Could you check a few things on this model? Use its own coordinates, in mm. A direction names the side the tool comes from. Give positions to 0.01 mm unless a question says otherwise; leave off trailing zeros. Loops run counter-clockwise (first coordinate to the right, second up) from the corner with the lowest first, then second, coordinate; pieces in that order, holes last. Notation, with made-up numbers: (-23.5, 71) -> (8.5, 71) arc R17 ccw to (8.5, 103) -> close; hole circle Ø7 at (77, 20). An arc over 180 degrees is marked (long way). Write each question's results on one line, items separated by ' | '. Start each with the question number.
Q1. Will these pins go through, and if not, where does the flat tip stop? P1, Ø4, axis at x = -31, y = -34.5, coming from the -Z side (3 decimals); P2, Ø6, axis at x = -31.75, z = -66.675, coming from the -Y side; P3, Ø8.5, axis at x = 34.75, z = 39.195, coming from the -Y side; P4, Ø20.5, axis at x = 0, z = 4.445, coming from the +Y side.
Q2. If we section it at C-C, the plane z = 11: List the corners of the cut face in (x, y) for me (3 decimals).
Q3. If we section it at A-A, the plane x = 0: List the corners of the cut face in (y, z) for me (3 decimals), plus the area to 3 significant figures.
Q4. If I drill on line 1 along X through (y, z) = (-38.5, 11) (3 decimals); line 2 along Y through (x, z) = (-9.5, 18.5); line 3 along Z through (x, y) = (-5.5, -17) (3 decimals), over which ranges is the centre line in solid material (lowest first)?
Q5. If we section it at B-B, the plane y = -6.5: List the corners of the cut face in (x, z) for me (3 decimals), plus the area to 3 significant figures.
Q6. If we section it at D-D, the plane y = -35: List the corners of the cut face in (x, z) for me (3 decimals), plus the area to 3 significant figures.
Q7. We'd pull the mould along X, two halves only. Please class faces 1 (the face through (-45.371, -51.333, 3.84)), 2 (the face through (3.81, 3.52, 16.56)), 3 (the face through (47.625, -31, -51)): released by +X, released by -X, zero draft, split by the parting line, or undercut.
Q8. Which directions (+Z, -Z, +X, -X, +Y, -Y) give clear straight access to the entire face, cutting with the end or side of a thin tool? Please do faces 4 (the face through (-37.28, 2.46, -31.85)), 5 (the face through (1, 2, -12)), 6 (the face through (-43.18, -41, 1)), 7 (the face through (-1, -30, -82)), 8 (the face through (45.43, -55.17, -35.09)).
from build123d import *

# Parameters (mm, degrees)
SKETCH1_W                      = 95.25
SKETCH1_H                      = 63.5
SKETCH1_H_2                    = 95.25
BOSS_EXTRUDE1_DEPTH            = 5
BOSS_EXTRUDE2_DEPTH            = 88.9
CUT_EXTRUDE1_REACH             = 170.812
CUT_EXTRUDE1_DIRECTION_2_REACH = 170.812
SKETCH4_R                      = 37.5
CUT_EXTRUDE2_DEPTH             = 2
CUT_EXTRUDE3_REACH             = 170.812
CUT_EXTRUDE3_DIRECTION_2_REACH = 170.812
FILLET1_R                      = 6.35
SKETCH6_W                      = 95.25
SKETCH6_H                      = 57.15
BOSS_EXTRUDE3_DEPTH            = 30
CUT_EXTRUDE4_REACH             = 136.485
SKETCH7_R                      = 2.665000004
CUT_EXTRUDE5_REACH             = 155.082
SKETCH8_R                      = 12.7
CUT_EXTRUDE6_REACH             = 152.067
SKETCH9_R                      = 3.25


with BuildPart() as part:
    # Sketch1 → Boss-Extrude1 (new body)
    with BuildSketch(Plane(origin=(0, 0, 0), x_dir=(1, 0, 0), z_dir=(0, 1, 0))):
        with Locations((0, 79.375)):
            Rectangle(SKETCH1_W, SKETCH1_H)
        Rectangle(SKETCH1_W, SKETCH1_H_2)
    extrude(amount=BOSS_EXTRUDE1_DEPTH)

    # Sketch2 → Boss-Extrude2 (add)
    with BuildSketch(Plane(origin=(0, 0, 0), x_dir=(-1, 0, 0), z_dir=(0, -1, 0))):
        Polygon((43.18, 38.735), (43.18, -47.625), (47.625, -47.625), (47.625, 53.975), (-47.625, 53.975), (-47.625, -47.625), (-43.18, -47.625), (-43.18, 38.735), align=None)
    extrude(amount=BOSS_EXTRUDE2_DEPTH)

    # Sketch3 → Cut-Extrude1 (cut, up to next)
    with BuildSketch(Plane.ZY.offset(-43.18), mode=Mode.PRIVATE) as cut_extrude1_sk1:
        Polygon((-38.735, -88.9), (47.625, -12.7), (47.625, -88.9), align=None)
    cut_extrude1_tool1 = extrude(cut_extrude1_sk1.sketch, amount=-CUT_EXTRUDE1_REACH, mode=Mode.PRIVATE) & part.part
    add(cut_extrude1_tool1.solids().sort_by_distance((43.18, -63.5, 18.838333))[0], mode=Mode.SUBTRACT)

    # Sketch3 → Cut-Extrude1 direction 2 (cut, up to next)
    with BuildSketch(Plane.ZY.offset(-43.18), mode=Mode.PRIVATE) as cut_extrude1_direction_2_sk1:
        Polygon((-38.735, -88.9), (47.625, -12.7), (47.625, -88.9), align=None)
    cut_extrude1_direction_2_tool1 = extrude(cut_extrude1_direction_2_sk1.sketch, amount=CUT_EXTRUDE1_DIRECTION_2_REACH, mode=Mode.PRIVATE) & part.part
    add(cut_extrude1_direction_2_tool1.solids().sort_by_distance((43.18, -63.5, 18.838333))[0], mode=Mode.SUBTRACT)

    # Sketch4 → Cut-Extrude2 (cut)
    with BuildSketch(Plane(origin=(0, 0, 0), x_dir=(-1, 0, 0), z_dir=(0, -1, 0))):
        with Locations(Location((0, -4.445, 0), (0, 0, 90))):
            Circle(SKETCH4_R)
    extrude(amount=-CUT_EXTRUDE2_DEPTH, mode=Mode.SUBTRACT)

    # Sketch5 → Cut-Extrude3 (cut, up to next)
    with BuildSketch(Plane(origin=(-43.18, 0, 0), x_dir=(0, 0, -1), z_dir=(1, 0, 0)), mode=Mode.PRIVATE) as cut_extrude3_sk1:
        Polygon((38.735, 0), (-33.225441849, 0), (38.735, -63.494507514), align=None)
    cut_extrude3_tool1 = extrude(cut_extrude3_sk1.sketch, amount=-CUT_EXTRUDE3_REACH, mode=Mode.PRIVATE) & part.part
    add(cut_extrude3_tool1.solids().sort_by_distance((-43.18, -21.164836, -14.748186))[0], mode=Mode.SUBTRACT)

    # Sketch5 → Cut-Extrude3 direction 2 (cut, up to next)
    with BuildSketch(Plane(origin=(-43.18, 0, 0), x_dir=(0, 0, -1), z_dir=(1, 0, 0)), mode=Mode.PRIVATE) as cut_extrude3_direction_2_sk1:
        Polygon((38.735, 0), (-33.225441849, 0), (38.735, -63.494507514), align=None)
    cut_extrude3_direction_2_tool1 = extrude(cut_extrude3_direction_2_sk1.sketch, amount=CUT_EXTRUDE3_DIRECTION_2_REACH, mode=Mode.PRIVATE) & part.part
    add(cut_extrude3_direction_2_tool1.solids().sort_by_distance((-43.18, -21.164836, -14.748186))[0], mode=Mode.SUBTRACT)

    # Fillet1
    fillet1_edges = [part.edges().sort_by_distance(p)[0] for p in [
        (45.4025, -63.494507514, -38.735),
        (45.4025, 0, 33.225441849),
        (-45.4025, 0, 33.225441849),
        (-45.4025, -63.494507514, -38.735),
    ]]
    fillet(fillet1_edges, radius=FILLET1_R)

    # Sketch6 → Boss-Extrude3 (add)
    with BuildSketch(Plane.XZ):
        with Locations((0, -82.55)):
            Rectangle(SKETCH6_W, SKETCH6_H)
    extrude(amount=BOSS_EXTRUDE3_DEPTH)

    # Sketch7 → Cut-Extrude4 (cut, up to next)
    with BuildSketch(Plane(origin=(0, -30, 0), x_dir=(-1, 0, 0), z_dir=(0, -1, 0)), mode=Mode.PRIVATE) as cut_extrude4_sk1:
        with Locations(Location((0, 97.872945695, 0), (0, 0, 90))):
            Circle(SKETCH7_R)
    cut_extrude4_tool1 = extrude(cut_extrude4_sk1.sketch, amount=-CUT_EXTRUDE4_REACH, mode=Mode.PRIVATE) & part.part
    # Sketch7 → Cut-Extrude4 (cut, up to next)
    with BuildSketch(Plane(origin=(0, -30, 0), x_dir=(-1, 0, 0), z_dir=(0, -1, 0)), mode=Mode.PRIVATE) as cut_extrude4_sk2:
        with Locations(Location((31.75, 66.675, 0), (0, 0, 90))):
            Circle(SKETCH7_R)
    cut_extrude4_tool2 = extrude(cut_extrude4_sk2.sketch, amount=-CUT_EXTRUDE4_REACH, mode=Mode.PRIVATE) & part.part
    # Sketch7 → Cut-Extrude4 (cut, up to next)
    with BuildSketch(Plane(origin=(0, -30, 0), x_dir=(-1, 0, 0), z_dir=(0, -1, 0)), mode=Mode.PRIVATE) as cut_extrude4_sk3:
        with Locations(Location((-31.75, 66.675, 0), (0, 0, 90))):
            Circle(SKETCH7_R)
    cut_extrude4_tool3 = extrude(cut_extrude4_sk3.sketch, amount=-CUT_EXTRUDE4_REACH, mode=Mode.PRIVATE) & part.part
    add(cut_extrude4_tool1.solids().sort_by_distance((0, -30, -97.872946))[0], mode=Mode.SUBTRACT)
    add(cut_extrude4_tool2.solids().sort_by_distance((-31.75, -30, -66.675))[0], mode=Mode.SUBTRACT)
    add(cut_extrude4_tool3.solids().sort_by_distance((31.75, -30, -66.675))[0], mode=Mode.SUBTRACT)

    # Sketch8 → Cut-Extrude5 (cut, up to next)
    with BuildSketch(Plane(origin=(0, 5, 0), x_dir=(1, 0, 0), z_dir=(0, 1, 0)), mode=Mode.PRIVATE) as cut_extrude5_sk1:
        with Locations(Location((0, -4.445, 0), (0, 0, 270))):
            Circle(SKETCH8_R)
    cut_extrude5_tool1 = extrude(cut_extrude5_sk1.sketch, amount=-CUT_EXTRUDE5_REACH, mode=Mode.PRIVATE) & part.part
    add(cut_extrude5_tool1.solids().sort_by_distance((0, 5, 4.445))[0], mode=Mode.SUBTRACT)

    # Sketch9 → Cut-Extrude6 (cut, up to next)
    with BuildSketch(Plane(origin=(0, 0, 0), x_dir=(-1, 0, 0), z_dir=(0, -1, 0)), mode=Mode.PRIVATE) as cut_extrude6_sk1:
        with Locations(Location((34.75, -39.195, 0), (0, 0, 90))):
            Circle(SKETCH9_R)
    cut_extrude6_tool1 = extrude(cut_extrude6_sk1.sketch, amount=-CUT_EXTRUDE6_REACH, mode=Mode.PRIVATE) & part.part
    # Sketch9 → Cut-Extrude6 (cut, up to next)
    with BuildSketch(Plane(origin=(0, 0, 0), x_dir=(-1, 0, 0), z_dir=(0, -1, 0)), mode=Mode.PRIVATE) as cut_extrude6_sk2:
        with Locations(Location((-34.75, -39.195, 0), (0, 0, 90))):
            Circle(SKETCH9_R)
    cut_extrude6_tool2 = extrude(cut_extrude6_sk2.sketch, amount=-CUT_EXTRUDE6_REACH, mode=Mode.PRIVATE) & part.part
    # Sketch9 → Cut-Extrude6 (cut, up to next)
    with BuildSketch(Plane(origin=(0, 0, 0), x_dir=(-1, 0, 0), z_dir=(0, -1, 0)), mode=Mode.PRIVATE) as cut_extrude6_sk3:
        with Locations(Location((34.396603139, 30.34702737, 0), (0, 0, 90))):
            Circle(SKETCH9_R)
    cut_extrude6_tool3 = extrude(cut_extrude6_sk3.sketch, amount=-CUT_EXTRUDE6_REACH, mode=Mode.PRIVATE) & part.part
    # Sketch9 → Cut-Extrude6 (cut, up to next)
    with BuildSketch(Plane(origin=(0, 0, 0), x_dir=(-1, 0, 0), z_dir=(0, -1, 0)), mode=Mode.PRIVATE) as cut_extrude6_sk4:
        with Locations(Location((-34.75, 30.305, 0), (0, 0, 90))):
            Circle(SKETCH9_R)
    cut_extrude6_tool4 = extrude(cut_extrude6_sk4.sketch, amount=-CUT_EXTRUDE6_REACH, mode=Mode.PRIVATE) & part.part
    add(cut_extrude6_tool1.solids().sort_by_distance((-34.75, 0, 39.195))[0], mode=Mode.SUBTRACT)
    add(cut_extrude6_tool2.solids().sort_by_distance((34.75, 0, 39.195))[0], mode=Mode.SUBTRACT)
    add(cut_extrude6_tool3.solids().sort_by_distance((-34.396603, 0, -30.347027))[0], mode=Mode.SUBTRACT)
    add(cut_extrude6_tool4.solids().sort_by_distance((34.75, 0, -30.305))[0], mode=Mode.SUBTRACT)


solid = part.part
Final values:
1) P1: stops at z = -53.975 | P2: stops at y = -30 | P3: stops at y = 0 | P4: passes through
2) outline: (-47.625, -45.016) -> (-43.18, -45.016) -> (-43.18, -19.611) -> (-47.625, -19.611) -> close; (-47.625, 0) -> (-36.923, 0) -> (-36.923, 2) -> (-10.878, 2) -> (-10.878, 5) -> (-47.625, 5) -> close; (10.878, 2) -> (36.923, 2) -> (36.923, 0) -> (47.625, 0) -> (47.625, 5) -> (10.878, 5) -> close; (43.18, -45.016) -> (47.625, -45.016) -> (47.625, -19.611) -> (43.18, -19.611) -> close
3) outline: (-88.9, -53.975) -> (-30, -53.975) -> (-30, -95.208) -> (5, -95.208) -> (5, -8.255) -> (2, -8.255) -> (2, -33.055) -> (0, -33.055) -> (0, -38.735) -> (-88.9, -38.735) -> close; (-30, -111.125) -> (5, -111.125) -> (5, -100.538) -> (-30, -100.538) -> close; (0, 41.945) -> (2, 41.945) -> (2, 17.145) -> (5, 17.145) -> (5, 47.625) -> (0, 47.625) -> close | area: 3,450 mm²
4) line 1: x = -47.625 to -43.18, 43.18 to 47.625 | line 2: y = 2 to 5 | line 3: z = -111.125 to -38.735
5) outline: (-47.625, -111.125) -> (47.625, -111.125) -> (47.625, -38.735) -> (-47.625, -38.735) -> close; (-47.625, 22.779) -> (-43.18, 22.779) -> (-43.18, 47.625) -> (-47.625, 47.625) -> close; (43.18, 22.779) -> (47.625, 22.779) -> (47.625, 47.625) -> (43.18, 47.625) -> close; hole circle Ø5.33 at (-31.75, -66.675); hole circle Ø5.33 at (0, -97.873); hole circle Ø5.33 at (31.75, -66.675) | area: 7,050 mm²
6) outline: (-47.625, -53.975) -> (47.625, -53.975) -> (47.625, -38.735) -> (-47.625, -38.735) -> close; (-47.625, -6.441) -> (-43.18, -6.441) -> (-43.18, 22.352) -> (-47.625, 22.352) -> close; (43.18, -6.441) -> (47.625, -6.441) -> (47.625, 22.352) -> (43.18, 22.352) -> close | area: 1,710 mm²
7) face 1: zero draft | face 2: undercut | face 3: released by +X
8) face 4: +Y, -Y | face 5: -Y | face 6: +Z, -Y | face 7: -Z, +X, -X, -Y | face 8: +X, -X
